Build history of the part. All positions in model axes, mm. Face numbers are marked on the shaded views. A direction names the side the tool comes from. Coordinates: 2 decimals unless noted, no trailing zeros. Order: outer loops, then holes, each group sorted by start corner. A loop starts at its lowest first (then second) coordinate and runs counter-clockwise, first axis right, second up. Notation, with made-up numbers: (-7, 24) -> (-2, 24) arc R31 ccw to (-2, 60) -> close; hole circle Ø5 at (-23, 65). An arc over 180 degrees is marked (long way). Write each question's results on one line, items separated by ' | '.
from build123d import *
from OCP.BRepFilletAPI import BRepFilletAPI_MakeChamfer

# Parameters (mm, degrees)
SKETCH_1_W          = 58
SKETCH_1_H          = 36
EXTRUDE_1_DEPTH     = 6
SKETCH_2_W          = 52.5
SKETCH_2_H          = 30.5
CUT_EXTRUDE_1_DEPTH = 5.2
FILLET_1_R          = 2
SKETCH_3_W          = 4
SKETCH_3_H          = 30.5
EXTRUDE_2_DEPTH     = 3.7
FILLET_2_R          = 4
CHAMFER_1_SIZE      = 2
SKETCH_4_W          = 11
SKETCH_4_H          = 5.2
CUT_EXTRUDE_2_DEPTH = 10
FILLET_3_R          = 0.2
CHAMFER_2_SIZE      = 0.2
CHAMFER_2_SIZE_2    = 0.141421356
M1_2X0_25_1_D       = 0.95
M1_2X0_25_1_DEPTH   = 3
M1_2X0_25_1_TIP     = 0.285408794


with BuildPart() as part:
    # 草图1 → 凸台-拉伸1 (new body)
    with BuildSketch(Plane.XY):
        Rectangle(SKETCH_1_W, SKETCH_1_H)
    extrude(amount=EXTRUDE_1_DEPTH)

    # 草图2 → 切除-拉伸1 (cut)
    with BuildSketch(Plane(origin=(0, 0, 0), x_dir=(-1, 0, 0), z_dir=(0, 0, -1))):
        Rectangle(SKETCH_2_W, SKETCH_2_H)
    extrude(amount=-CUT_EXTRUDE_1_DEPTH, mode=Mode.SUBTRACT)

    # 圆角1
    fillet_1_edges = [part.edges().sort_by_distance(p)[0] for p in [
        (29, -18, 3),
        (-29, -18, 3),
        (-29, 18, 3),
        (29, 18, 3),
    ]]
    fillet(fillet_1_edges, radius=FILLET_1_R)

    # 草图3 → 凸台-拉伸2 (add)
    with BuildSketch(Plane(origin=(0, 0, 5.2), x_dir=(-1, 0, 0), z_dir=(0, 0, -1))):
        with Locations((13.25, 0)):
            Rectangle(SKETCH_3_W, SKETCH_3_H)
    extrude(amount=EXTRUDE_2_DEPTH)

    # 圆角2
    fillet_2_edges = [part.edges().sort_by_distance(p)[0] for p in [
        (-15.25, -15.25, 3.35),
        (-15.25, 15.25, 3.35),
        (-11.25, 15.25, 3.35),
        (-11.25, -15.25, 3.35),
    ]]
    fillet(fillet_2_edges, radius=FILLET_2_R)

    # 倒角1
    chamfer_1_edges = [part.edges().sort_by_distance(p)[0] for p in [
        (-29, 0, 6),
        (0, 18, 6),
        (29, 0, 6),
        (0, -18, 6),
        (28.414213562, -17.414213562, 6),
        (28.414213562, 17.414213562, 6),
        (-28.414213562, -17.414213562, 6),
        (-28.414213562, 17.414213562, 6),
    ]]
    chamfer(chamfer_1_edges, length=CHAMFER_1_SIZE)

    # 草图4 → 切除-拉伸2 (cut)
    with BuildSketch(Plane(origin=(0, 18, 0), x_dir=(1, 0, 0), z_dir=(0, 1, 0))):
        with Locations((19.5, -2.6)):
            Rectangle(SKETCH_4_W, SKETCH_4_H)
    extrude(amount=-CUT_EXTRUDE_2_DEPTH, mode=Mode.SUBTRACT)

    # 圆角3
    fillet_3_edges = [part.edges().sort_by_distance(p)[0] for p in [
        (-26.25, 15.25, 2.6),
        (-26.25, -15.25, 2.6),
        (26.25, -15.25, 2.6),
        (26.25, 15.25, 2.6),
    ]]
    fillet(fillet_3_edges, radius=FILLET_3_R)

    # 倒角2
    chamfer_2_edges_1 = [part.edges().sort_by_distance(p)[0] for p in [
        (14, 17.4, 4.6),
        (25, 17.4, 4.6),
        (25, 18, 2),
        (14, 18, 2),
    ]]
    chamfer_2_edges_2 = [part.edges().sort_by_distance(p)[0] for p in [
        (19.5, 16.8, 5.2),
    ]]
    chamfer_2_side_2 = [part.faces().sort_by_distance(p)[0] for p in [
        (19.5, 16.797171573, 5.2),
    ]]
    chamfer_2 = BRepFilletAPI_MakeChamfer(part.part.solid().wrapped)
    for e in chamfer_2_edges_1:
        chamfer_2.Add(CHAMFER_2_SIZE - 0.0001, e.wrapped)
    for e in chamfer_2_edges_2:
        chamfer_2.Add(CHAMFER_2_SIZE_2 - 0.0001, CHAMFER_2_SIZE - 0.0001, e.wrapped, chamfer_2_side_2[0].wrapped)
    add(Compound.cast(chamfer_2.Shape()), mode=Mode.REPLACE)  # a hair under: the kernel refuses the full size

    # M1.2x0.25 螺纹孔1
    with Locations(Plane(origin=(27.5, 16.5, 0), x_dir=(-1, 0, 0), z_dir=(0, 0, -1))):
        with Locations((0, 0), (0, -33), (55, -33), (55, 0)):
            Hole(M1_2X0_25_1_D / 2, depth=M1_2X0_25_1_DEPTH)
            with Locations((0, 0, -(M1_2X0_25_1_DEPTH + M1_2X0_25_1_TIP / 2))):  # 118° drill point
                Cone(0, M1_2X0_25_1_D / 2, M1_2X0_25_1_TIP, mode=Mode.SUBTRACT)


solid = part.part
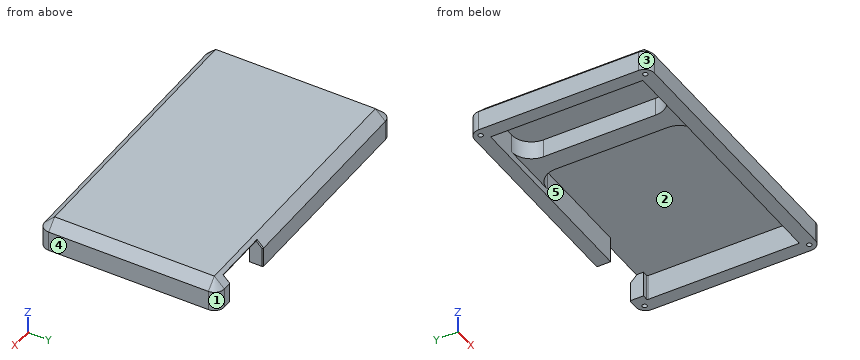
Item 1: Slice it at B-B, the plane x = -21. List the corners of the cut face in (y, z).
Answer:
outline: (-18, 0) -> (-15.25, 0) -> (-15.25, 5.2) -> (15.25, 5.2) -> (15.25, 0) -> (18, 0) -> (18, 4) -> (16, 6) -> (-16, 6) -> (-18, 4) -> close
Item 2: Slice it at C-C, the plane y = -2. List the corners of the cut face in (x, z), and give its area (3 significant figures).
Answer:
outline: (-29, 0) -> (-26.25, 0) -> (-26.25, 5.2) -> (-15.25, 5.2) -> (-15.25, 1.5) -> (-11.25, 1.5) -> (-11.25, 5.2) -> (26.25, 5.2) -> (26.25, 0) -> (29, 0) -> (29, 4) -> (27, 6) -> (-27, 6) -> (-29, 4) -> close | area: 85.8 mm^2
Item 3: Pin check, flat tips, straight feed: pin 1 (0.8 mm diameter, centred on y = 16.5, z = 1.5, fed in from -X); pin 2 (8 mm diameter, centred on x = -9.5, y = -2.5, fed in from -Z); pin 3 (16 mm diameter, centred on x = 16, y = -7, fed in from -Z). Stop position of each tip, or through.
Answer:
pin 1: stops at x = -29 | pin 2: stops at z = 1.5 | pin 3: stops at z = 5.2
Item 4: Slice it at A-A, the plane z = 2.25. State how many separate pieces and enclosed holes the cut face has, and give its area (3 significant figures).
Answer:
separate pieces: 1 | enclosed holes: 5 | area: 586 mm^2
Item 5: Pull direction Y, two halves, no side cores. Call the marked faces 1, 2 and 3: released by +Y, released by -Y, zero draft, split by the parting line, or undercut.
Answer:
face 1: released by +Y | face 2: undercut | face 3: released by -Y
Item 6: Drill centre lines: line 1 (Y direction, x = 7.5, z = 1); line 2 (X direction, y = 10.5, z = 2); line 3 (X direction, y = 11.5, z = 1.25). Where is each one in solid material? Low to high. Write a range as from..to.
Answer:
line 1: y = -18..-15.25, 15.25..18 | line 2: x = -29..-26.25, -15.25..-11.25, 26.25..29 | line 3: x = -29..-26.25, 26.25..29
Item 7: Tool access for the marked faces 4 and 5: list every direction of +Z, -Z, +X, -X, +Y, -Y with a clear straight run to the whole face (end or side of a thin tool).
Answer:
face 4: +Z, -Z, +X, +Y, -Y | face 5: -Z
